Design review of the part built by this model. Coordinates are the model's own, in mm. Face numbers are marked on the shaded views. Coordinates: 2 decimals unless noted, no trailing zeros. Write each loop counter-clockwise with the first axis right and the second up, starting at its lowest first coordinate (ties: lowest second). Pieces come first, ordered by that corner, then holes.
Q1. Take a section at D-D (y = 11). Give the boundary of the cut face in (x, z).
Q2. Insertion check: pin 1 (1 mm diameter, centred on x = 5, z = 43.5, fed in from +Y); pin 2 (8 mm diameter, centred on x = 17, y = 2, fed in from +Z); pin 3 (1.5 mm diameter, centred on y = 6.5, z = -4.5, fed in from -X); pin 4 (2.5 mm diameter, centred on x = -15, z = -8.55, fed in from -Y). Each pin has a flat end and moves straight along its axis. Give the tip position at first contact, or say it passes through.
Q3. Mouldability with a two-part tool opening along Z and no side actions: class the marked faces 1 and 2 as pulls with the +Z half, pulls with the -Z half, needs draft (parallel to the pull), parting line crosses it, or undercut.
Q4. Take a section at B-B (x = -15). Give the boundary of the cut face in (y, z).
Q5. Take a section at A-A (z = 8.55). Give the boundary of the cut face in (x, y), and give its area (3 significant figures).
Q6. Take a section at C-C (y = 7). Give the boundary of the cut face in (x, z), and give its area (3 significant figures).
Q7. For probe 1 along X at (y, z) = (2.05, -8.55); probe 2 along Z at (x, y) = (-15, 3.6); probe 3 along Y at (x, z) = (0, -33.5), list the stretches that pass through material, from the lowest coordinate up.
```python
from build123d import *

# Parameters (mm, degrees)
SKETCH_1_R      = 1.5
EXTRUDE_1_DEPTH = 5
SKETCH_2_R      = 3.5
EXTRUDE_2_DEPTH = 10
EXTRUDE_3_DEPTH = 5
SKETCH_4_R      = 1
EXTRUDE_4_DEPTH = 3


with BuildPart() as part:
    # 草图1 → 凸台-拉伸1 (new body)
    with BuildSketch(Plane(origin=(0, 0, 0), x_dir=(1, 0, 0), z_dir=(0, 1, 0))):
        with BuildLine():
            Line((-39.038561358, -22.382822144), (-39.038561358, 22.382822144))
            ThreePointArc((-39.038561358, 22.382822144), (-8.857541047, 44.119655105), (27.374530931, 35.716033603))
            Line((27.374530931, 35.716033603), (27.374530931, -35.716033603))
            ThreePointArc((27.374530931, -35.716033603), (-8.857541047, -44.119655105), (-39.038561358, -22.382822144))
        make_face()
        with Locations((-15, 8.55)):
            Circle(SKETCH_1_R, mode=Mode.SUBTRACT)
        with Locations((-15, -8.55)):
            Circle(SKETCH_1_R, mode=Mode.SUBTRACT)
    extrude(amount=EXTRUDE_1_DEPTH)

    # 草图2 → 凸台-拉伸2 (add)
    with BuildSketch(Plane(origin=(0, 5, 0), x_dir=(1, 0, 0), z_dir=(0, 1, 0))):
        with Locations((15, -8.55)):
            Circle(SKETCH_2_R)
    extrude(amount=EXTRUDE_2_DEPTH)

    # 草图3 → 凸台-拉伸3 (add)
    with BuildSketch(Plane(origin=(0, 5, 0), x_dir=(1, 0, 0), z_dir=(0, 1, 0))):
        with BuildLine():
            ThreePointArc((0, -45), (13.278516311, -42.996290591), (25.374530931, -37.163600203))
            Line((25.374530931, -37.163600203), (25.374530931, -33.46839076))
            ThreePointArc((25.374530931, -33.46839076), (13.385208031, -39.810001331), (0, -42))
            Line((0, -42), (0, -45))
        make_face()
        with BuildLine():
            Line((25.374530931, -33.46839076), (25.374530931, -37.163600203))
            ThreePointArc((25.374530931, -37.163600203), (26.384460277, -36.453535575), (27.374530931, -35.716033603))
            Line((27.374530931, -35.716033603), (27.374530931, -31.853336659))
            ThreePointArc((27.374530931, -31.853336659), (26.386890339, -32.676168965), (25.374530931, -33.46839076))
        make_face()
        with BuildLine():
            Line((25.374530931, 33.46839076), (25.374530931, -33.46839076))
            ThreePointArc((25.374530931, -33.46839076), (26.386890339, -32.676168965), (27.374530931, -31.853336659))
            Line((27.374530931, -31.853336659), (27.374530931, 31.853336659))
            ThreePointArc((27.374530931, 31.853336659), (26.386890339, 32.676168965), (25.374530931, 33.46839076))
        make_face()
        with BuildLine():
            Line((25.374530931, 37.163600203), (25.374530931, 33.46839076))
            ThreePointArc((25.374530931, 33.46839076), (26.386890339, 32.676168965), (27.374530931, 31.853336659))
            Line((27.374530931, 31.853336659), (27.374530931, 35.716033603))
            ThreePointArc((27.374530931, 35.716033603), (26.384460277, 36.453535575), (25.374530931, 37.163600203))
        make_face()
        with BuildLine():
            ThreePointArc((0, 42), (13.385208031, 39.810001331), (25.374530931, 33.46839076))
            Line((25.374530931, 33.46839076), (25.374530931, 37.163600203))
            ThreePointArc((25.374530931, 37.163600203), (13.278516311, 42.996290591), (0, 45))
            Line((0, 45), (0, 42))
        make_face()
    extrude(amount=EXTRUDE_3_DEPTH)

    # 草图4 → 凸台-拉伸4 (add)
    with BuildSketch(Plane(origin=(0, 10, 0), x_dir=(1, 0, 0), z_dir=(0, 1, 0))):
        with Locations((26.074530931, -34.848835383)):
            Circle(SKETCH_4_R)
        with Locations((5.074530931, -43.226977996)):
            Circle(SKETCH_4_R)
        with Locations((26.074530931, 34.848835383)):
            Circle(SKETCH_4_R)
        with Locations((5.074530931, 43.226977996)):
            Circle(SKETCH_4_R)
    extrude(amount=EXTRUDE_4_DEPTH)


solid = part.part
```
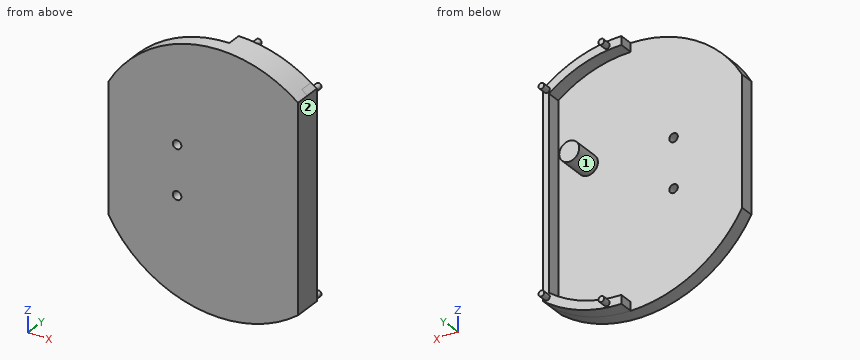
Response:
1. outline: circle Ø2 at (5.07, -43.23); circle Ø2 at (5.07, 43.23); circle Ø7 at (15, 8.55); circle Ø2 at (26.07, -34.85); circle Ø2 at (26.07, 34.85)
2. pin 1: stops at y = 13
2. pin 2: stops at z = 43.08
2. pin 3: stops at x = 25.37
2. pin 4: passes through
3. face 1: undercut
3. face 2: needs draft
4. outline: (0, -42.43) - (5, -42.43) - (5, -10.05) - (0, -10.05) - close; (0, -7.05) - (5, -7.05) - (5, 7.05) - (0, 7.05) - close; (0, 10.05) - (5, 10.05) - (5, 42.43) - (0, 42.43) - close
5. outline: (-39.04, 0) - (-16.5, 0) - (-16.5, 5) - (-39.04, 5) - close; (-13.5, 0) - (27.37, 0) - (27.37, 10) - (25.37, 10) - (25.37, 5) - (18.5, 5) - (18.5, 15) - (11.5, 15) - (11.5, 5) - (-13.5, 5) - close
5. area: 397 mm2
6. outline: (0, -45) arc R45 ccw to (27.37, -35.72) - (27.37, 35.72) arc R45 ccw to (0, 45) - (0, 42) arc R42 cw to (25.37, 33.47) - (25.37, -33.47) arc R42 cw to (0, -42) - close; circle Ø7 at (15, 8.55)
6. area: 347 mm2
7. probe 1: x = -39.04 to -16.5, -13.5 to 27.37
7. probe 2: z = -42.43 to -10.05, -7.05 to 7.05, 10.05 to 42.43
7. probe 3: y = 0 to 5
